Can you work these out from the model? Positions are in its coordinate system, mm. Face numbers are marked on the shaded views. A direction names the side the tool comes from. Give positions to 0.01 mm unless a question says otherwise; leave off trailing zeros. Loops run counter-clockwise (first coordinate to the right, second up) from the corner with the lowest first, then second, coordinate; pieces in that order, holes last. Notation, with made-up numbers: M 74.5,19.25 L 128.5,19.25 A14 ccw 128.5,42.25 Z; hole C -39.75,30.25 d10. An arc over 180 degrees is marked long. Put each result on its own line as item: value. Start each with the question number.
1) Imagine slicing it at C-C (y = 50). Write out the boundary of the cut face in (x, z).
2) For P1, Ø2, axis at y = 43.5, z = 12, coming from the +X side, with a flat end and sliding along its axis, tell me the tip position at first contact or that it passes through.
3) Imagine slicing it at B-B (x = 55.5). Write out the boundary of the cut face in (y, z).
4) If we mould it in two halves opening along Z, with no side actions, what happens to the marked faces 1, 2 and 3? For each: +Z half, -Z half, draft (parallel to the pull), parting line (faces both ways), or undercut.
5) Imagine slicing it at A-A (z = 8). Write out the boundary of the cut face in (x, y).
6) For the marked faces 4 and 5, which set-ups out of +Z, -Z, +X, -X, +Y, -Y let a thin tool reach every point of the face, with its end or its side?
7) Imagine slicing it at D-D (z = 2.25). Write out the boundary of the cut face in (x, y), then the cut area to 3 significant figures.
8) Please list where these lines run through material, in increasing order: line 1 along X through (y, z) = (32.25, 7.75); line 2 along Z through (x, y) = (58.75, 45.25); line 3 along X through (y, z) = (38.5, 12.5). Write a range as from..to.
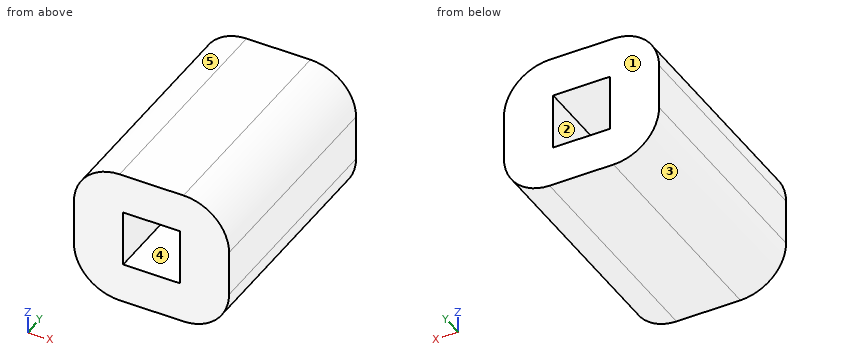
from build123d import *

# Parameters (mm, degrees)
SKETCH1_W           = 17
SKETCH1_H           = 25
BOSS_EXTRUDE1_DEPTH = 15
SKETCH2_W           = 6.2
SKETCH2_H           = 6.2
CUT_EXTRUDE1_DEPTH  = 3.25
SKETCH3_W           = 6.2
SKETCH3_H           = 6.2
CUT_EXTRUDE2_DEPTH  = 3.25
FILLET1_R           = 5
SKETCH6_W           = 6.2
SKETCH6_H           = 6.2
CUT_EXTRUDE3_DEPTH  = 71.704212299


with BuildPart() as part:
    # Sketch1 → Boss-Extrude1 (new body)
    with BuildSketch(Plane.XY):
        with Locations((57.082186124, 39.41449257)):
            Rectangle(SKETCH1_W, SKETCH1_H)
    extrude(amount=BOSS_EXTRUDE1_DEPTH)

    # Sketch2 → Cut-Extrude1 (cut)
    with BuildSketch(Plane.XZ.offset(-26.91449257)):
        with Locations((57.082186124, 7.5)):
            Rectangle(SKETCH2_W, SKETCH2_H)
    extrude(amount=-CUT_EXTRUDE1_DEPTH, mode=Mode.SUBTRACT)

    # Sketch3 → Cut-Extrude2 (cut)
    with BuildSketch(Plane(origin=(0, 51.91449257, 0), x_dir=(1, 0, 0), z_dir=(0, 1, 0))):
        with Locations((57.082186124, -7.5)):
            Rectangle(SKETCH3_W, SKETCH3_H)
    extrude(amount=-CUT_EXTRUDE2_DEPTH, mode=Mode.SUBTRACT)

    # Fillet1
    fillet1_edges = [part.edges().sort_by_distance(p)[0] for p in [
        (48.582186124, 39.41449257, 15),
        (65.582186124, 39.41449257, 15),
        (48.582186124, 39.41449257, 0),
        (65.582186124, 39.41449257, 0),
    ]]
    fillet(fillet1_edges, radius=FILLET1_R)

    # Sketch6 → Cut-Extrude3 (cut, through all)
    with BuildSketch(Plane(origin=(0, 48.66449257, 0), x_dir=(1, 0, 0), z_dir=(0, 1, 0))):
        with Locations((57.082186124, -7.5)):
            Rectangle(SKETCH6_W, SKETCH6_H)
    extrude(amount=-CUT_EXTRUDE3_DEPTH, mode=Mode.SUBTRACT)


solid = part.part
Recorded:
1. outline: M 48.58,5 A5 ccw 53.58,0 L 60.58,0 A5 ccw 65.58,5 L 65.58,10 A5 ccw 60.58,15 L 53.58,15 A5 ccw 48.58,10 Z; hole M 53.98,4.4 L 60.18,4.4 L 60.18,10.6 L 53.98,10.6 Z
2. P1: x = 65.48
3. outline: M 26.91,0 L 51.91,0 L 51.91,4.4 L 26.91,4.4 Z; M 26.91,10.6 L 51.91,10.6 L 51.91,15 L 26.91,15 Z
4. face 1: draft
4. face 2: undercut
4. face 3: -Z half
5. outline: M 48.58,26.91 L 53.98,26.91 L 53.98,51.91 L 48.58,51.91 Z; M 60.18,26.91 L 65.58,26.91 L 65.58,51.91 L 60.18,51.91 Z
6. face 4: +Y, -Y
6. face 5: +Z, -X, +Y, -Y
7. outline: M 49.41,26.91 L 64.76,26.91 L 64.76,51.91 L 49.41,51.91 Z
7. area: 384 mm²
8. line 1: 48.58..53.98, 60.18..65.58
8. line 2: 0..4.4, 10.6..15
8. line 3: 49.25..64.91
